```python
from build123d import *

# Parameters (mm, degrees)
SKETCH1_W           = 25.4
SKETCH1_H           = 17.78
BOSS_EXTRUDE1_DEPTH = 0.79375
SKETCH2_W           = 4.2545
SKETCH2_H           = 6.0325
BOSS_EXTRUDE2_DEPTH = 2.921
SKETCH3_R           = 1.27
CUT_EXTRUDE1_DEPTH  = 16.775117781
FILLET1_R           = 2.54


with BuildPart() as part:
    # Sketch1 → Boss-Extrude1 (new, symmetric)
    with BuildSketch(Plane.XY):
        Rectangle(SKETCH1_W, SKETCH1_H)
    extrude(amount=BOSS_EXTRUDE1_DEPTH, both=True)

    # Sketch2 → Boss-Extrude2 (add)
    with BuildSketch(Plane.XY.offset(0.79375)):
        with Locations((10.57275, 0)):
            Rectangle(SKETCH2_W, SKETCH2_H)
        with Locations((-10.57275, 0)):
            Rectangle(SKETCH2_W, SKETCH2_H)
    extrude(amount=BOSS_EXTRUDE2_DEPTH)

    # Sketch3 → Cut-Extrude1 (cut, through all)
    with BuildSketch(Plane.XY.offset(0.79375)):
        with Locations((-10.16, 6.35)):
            Circle(SKETCH3_R)
        with Locations((-10.16, -6.35)):
            Circle(SKETCH3_R)
        with Locations(Location((10.16, -6.35, 0), (0, 0, 180))):
            Circle(SKETCH3_R)
        with Locations(Location((10.16, 6.35, 0), (0, 0, 180))):
            Circle(SKETCH3_R)
    extrude(amount=-CUT_EXTRUDE1_DEPTH, mode=Mode.SUBTRACT)

    # Fillet1
    fillet1_edges = [part.edges().sort_by_distance(p)[0] for p in [
        (12.7, -8.89, 0),
        (-12.7, -8.89, 0),
        (-12.7, 8.89, 0),
        (12.7, 8.89, 0),
    ]]
    fillet(fillet1_edges, radius=FILLET1_R)


solid = part.part
```
Build history of the part. All positions in model axes, mm. A direction names the side the tool comes from. Give positions to 0.01 mm unless a question says otherwise; leave off trailing zeros. Loops run counter-clockwise (first coordinate to the right, second up) from the corner with the lowest first, then second, coordinate; pieces in that order, holes last. Notation, with made-up numbers: (-32.5, 52.25) -> (11.5, 52.25) arc R30 ccw to (11.5, 77.25) -> close; hole circle Ø10 at (46.5, -36). An arc over 180 degrees is marked (long way). One line per question, with ' | ' between items. Start each with the question number.
1) Cut at A-A (z = -0.4). Give the cut face in (x, y).
2) Cut at D-D (x = -0.25). Give the cut face in (y, z), plus the area to 3 significant figures.
3) Pin check, flat tips, straight feed: pin 1 (1.5 mm diameter, centred on x = 11.5, z = 2.5, fed in from -Y); pin 2 (0.9 mm diameter, centred on x = 10, z = 3, fed in from +Y); pin 3 (3.5 mm diameter, centred on x = -10.16, y = 6.35, fed in from +Z). Stop position of each tip, or through.
4) 3-axis set-ups, long thin cutter, end or side, ignore diameter. For faces 1 (the flat face through (-8.446, 0, 2)), 2 (the flat face through (11, 3.016, 2)), 3 (the flat face through (11, -3.016, 2)): which of +Z, -Z, +X, -X, +Y, -Y reach the whole face in a straight line?
5) Probe L1, parallel to Y at x = 10.16, z = 0.3; L2, parallel to X at y = -0.5, z = 2.15; L3, parallel to Z at x = 6, y = -3.5. List the from-to ranges inside material, lowest first.
6) Cut at C-C (z = 2.5). Give the cut face in (x, y), plus the area to 3 significant figures.
7) Two-plate mould, pull along X, no slides. Class faces 4 (the flat face through (11, 0, 3.715)), 5 (the flat face through (-12.7, 0, 1)), 6 (the cylindrical face through (11.9, 8.2, 0)), 7 (the cylindrical face through (8.95, -6.73, 0.01)): released by +X, released by -X, zero draft, split by the parting line, or undercut.
8) Cut at B-B (y = 1.25). Give the cut face in (x, z).
Return value:
1) outline: (-12.7, -6.35) arc R2.54 ccw to (-10.16, -8.89) -> (10.16, -8.89) arc R2.54 ccw to (12.7, -6.35) -> (12.7, 6.35) arc R2.54 ccw to (10.16, 8.89) -> (-10.16, 8.89) arc R2.54 ccw to (-12.7, 6.35) -> close; hole circle Ø2.54 at (-10.16, -6.35); hole circle Ø2.54 at (-10.16, 6.35); hole circle Ø2.54 at (10.16, -6.35); hole circle Ø2.54 at (10.16, 6.35)
2) outline: (-8.89, -0.79) -> (8.89, -0.79) -> (8.89, 0.79) -> (-8.89, 0.79) -> close | area: 28.2 mm^2
3) pin 1: y = -3.02 | pin 2: y = 3.02 | pin 3: z = 0.79
4) face 1: +Z, +Y, -Y | face 2: +Z, +X, -X, +Y | face 3: +Z, +X, -X, -Y
5) L1: -8.89 to -7.62, -5.08 to 5.08, 7.62 to 8.89 | L2: -12.7 to -8.45, 8.45 to 12.7 | L3: -0.79 to 0.79
6) outline: (-12.7, -3.02) -> (-8.45, -3.02) -> (-8.45, 3.02) -> (-12.7, 3.02) -> close; (8.45, -3.02) -> (12.7, -3.02) -> (12.7, 3.02) -> (8.45, 3.02) -> close | area: 51.3 mm^2
7) face 4: zero draft | face 5: released by -X | face 6: released by +X | face 7: undercut
8) outline: (-12.7, -0.79) -> (12.7, -0.79) -> (12.7, 3.71) -> (8.45, 3.71) -> (8.45, 0.79) -> (-8.45, 0.79) -> (-8.45, 3.71) -> (-12.7, 3.71) -> close
